```python
from build123d import *

# Parameters (mm, degrees)
BOSS_EXTRUDE1_DEPTH = 50
SKETCH2_W           = 1500
SKETCH2_H           = 450
BOSS_EXTRUDE2_DEPTH = 10
LPATTERN1_COUNT     = 2
LPATTERN1_PITCH     = 1450
LPATTERN2_COUNT     = 3
LPATTERN2_PITCH     = 490
CUT_EXTRUDE1_REACH  = 1685.38
SKETCH3_R           = 35


with BuildPart() as part:
    # Sketch1 → Boss-Extrude1 (new body)
    with BuildSketch(Plane(origin=(0, 0, 0), x_dir=(0, 0, -1), z_dir=(1, 0, 0))):
        with BuildLine():
            Line((-720, -75), (720, -75))
            ThreePointArc((720, -75), (741.213203436, -66.213203436), (750, -45))
            Line((750, -45), (750, 45))
            ThreePointArc((750, 45), (741.213203436, 66.213203436), (720, 75))
            Line((720, 75), (-720, 75))
            ThreePointArc((-720, 75), (-741.213203436, 66.213203436), (-750, 45))
            Line((-750, 45), (-750, -45))
            ThreePointArc((-750, -45), (-741.213203436, -66.213203436), (-720, -75))
        make_face()
    boss_extrude1 = extrude(amount=BOSS_EXTRUDE1_DEPTH)

    # Sketch2 → Boss-Extrude2 (add)
    with BuildSketch(Plane(origin=(0, 75, 0), x_dir=(1, 0, 0), z_dir=(0, 1, 0))):
        with Locations((754.674039581, 490.104243835)):
            Rectangle(SKETCH2_W, SKETCH2_H)
    boss_extrude2 = extrude(amount=BOSS_EXTRUDE2_DEPTH)

    # LPattern1: Boss-Extrude1 ×2
    with Locations(*[(i * LPATTERN1_PITCH, 0, 0) for i in range(1, LPATTERN1_COUNT)]):
        add(boss_extrude1)

    # LPattern2: Boss-Extrude2 ×3
    with Locations(*[(0, 0, i * LPATTERN2_PITCH) for i in range(1, LPATTERN2_COUNT)]):
        add(boss_extrude2)

    # Cut-Extrude1: up to this face of the body (flat: up to its plane)
    cut_extrude1_end = Plane(part.part.faces().sort_by_distance((1500, 0, 0))[0])
    # Sketch3 → Cut-Extrude1 (cut, up to the picked face)
    with BuildSketch(Plane.ZY, mode=Mode.PRIVATE) as cut_extrude1_sk1:
        with Locations((-700, 0)):
            Circle(SKETCH3_R)
    cut_extrude1_tool1 = split(extrude(cut_extrude1_sk1.sketch, amount=-CUT_EXTRUDE1_REACH, mode=Mode.PRIVATE), bisect_by=cut_extrude1_end, keep=Keep.BOTH, mode=Mode.PRIVATE)
    # Sketch3 → Cut-Extrude1 (cut, up to the picked face)
    with BuildSketch(Plane.ZY, mode=Mode.PRIVATE) as cut_extrude1_sk2:
        with Locations((700, 0)):
            Circle(SKETCH3_R)
    cut_extrude1_tool2 = split(extrude(cut_extrude1_sk2.sketch, amount=-CUT_EXTRUDE1_REACH, mode=Mode.PRIVATE), bisect_by=cut_extrude1_end, keep=Keep.BOTH, mode=Mode.PRIVATE)
    add(cut_extrude1_tool1.solids().sort_by(Axis((0, 0, -700), (1, 0, 0)))[0], mode=Mode.SUBTRACT)
    add(cut_extrude1_tool2.solids().sort_by(Axis((0, 0, 700), (1, 0, 0)))[0], mode=Mode.SUBTRACT)


solid = part.part
```
Work out the finished part from the listing and answer in its coordinate system (mm). A direction names the side the tool comes from. Give positions to 0.01 mm unless a question says otherwise; leave off trailing zeros. Order: outer loops, then holes, each group sorted by start corner. A loop starts at its lowest first (then second) coordinate and runs counter-clockwise, first axis right, second up. Notation, with made-up numbers: (-28, 17) - (5, 17) arc R28 cw to (5, 38) - close; hole circle Ø2 at (53.25, 36). An arc over 180 degrees is marked (long way). One line per item, written item: value. Start each with the question number.
1. For a pull along Y with two mould halves and no side action, classify faces 4 (the face through (1475, -1, -750)), 5 (the face through (1475, -75, 10)), 6 (the face through (24.65, 10.513, -666.616)), 7 (the face through (744, 85, -493)) as released by +Y, released by -Y, zero draft, split by the parting line, or undercut.
2. Section B-B, the plane y = 0 is taken. Write down the section's boundary in (x, z).
3. Section A-A, the plane x = 1251.5 is taken. Write down the section's boundary in (y, z), then the cut area to 3 significant figures.
4. Each of these flat-tipped pins is pushed along its axis until it touches: pin 1 Ø12 at (y, z) = (37, 550) entering from +X; pin 2 Ø12 at (x, z) = (1468, -240) entering from +Y; pin 3 Ø2 at (x, z) = (762.5, -122) entering from -Y. Where does it stop, or does it pass through?
5. Consider line 1 (X direction, y = -56.5, z = -435.5); line 2 (Y direction, x = 1483, z = 700); line 3 (Y direction, x = 1230, z = 446). Determine where each line is inside the solid, lowest interval first.
6. Section C-C, the plane z = 246.5 is taken. Write down the section's boundary in (x, y).
7. Which of the six approach directions +Z, -Z, +X, -X, +Y, -Y give full straight-line access (tool end or side, diameter ignored) to faces 1 (the face through (744, 85, 487)), 2 (the face through (1475, 75, -245)), 3 (the face through (50, 1, 10))?
8. Section D-D, the plane z = 510.5 is taken. Write down the section's boundary in (x, y).
Filled sheet:
1. face 4: zero draft
1. face 5: released by -Y
1. face 6: undercut
1. face 7: released by +Y
2. outline: (0, -750) - (50, -750) - (50, -735) - (0, -735) - close; (0, -665) - (50, -665) - (50, 665) - (0, 665) - close; (0, 735) - (50, 735) - (50, 750) - (0, 750) - close; (1450, -750) - (1500, -750) - (1500, -735) - (1450, -735) - close; (1450, -665) - (1500, -665) - (1500, 665) - (1450, 665) - close; (1450, 735) - (1500, 735) - (1500, 750) - (1450, 750) - close
3. outline: (75, -715.1) - (85, -715.1) - (85, -265.1) - (75, -265.1) - close; (75, -225.1) - (85, -225.1) - (85, 224.9) - (75, 224.9) - close; (75, 264.9) - (85, 264.9) - (85, 714.9) - (75, 714.9) - close
3. area: 13,500 mm²
4. pin 1: x = 1500
4. pin 2: y = 75
4. pin 3: y = 75
5. line 1: 0 to 50, 1450 to 1500
5. line 2: -75 to -35, 35 to 85
5. line 3: 75 to 85
6. outline: (0, -75) - (50, -75) - (50, 75) - (0, 75) - close; (1450, -75) - (1500, -75) - (1500, 75) - (1450, 75) - close
7. face 1: +Z, -Z, +X, -X, +Y
7. face 2: +X, -X, +Y
7. face 3: +Z, -Z, -Y
8. outline: (0, -75) - (50, -75) - (50, 75) - (1450, 75) - (1450, -75) - (1500, -75) - (1500, 75) - (1504.67, 75) - (1504.67, 85) - (4.67, 85) - (4.67, 75) - (0, 75) - close
